Here's how the part is built. I have some questions about the finished solid (model axes, mm). A direction names the side the tool comes from. Give positions to 0.01 mm unless a question says otherwise; leave off trailing zeros. Loops run counter-clockwise (first coordinate to the right, second up) from the corner with the lowest first, then second, coordinate; pieces in that order, holes last. Notation, with made-up numbers: (21.5, 0.25) -> (73.5, 0.25) arc R22 cw to (73.5, 27.25) -> close; hole circle Ø3 at (88.5, -31.5). An arc over 180 degrees is marked (long way). Answer in a Markdown table with one row per item. Add a question column.
Item 1: If we section it at B-B (y = 0): Write out the boundary of the cut face in (x, z).
Item 2: If we section it at C-C (z = 10.5): Write out the boundary of the cut face in (x, y).
Item 3: If we section it at A-A (x = 0): Write out the boundary of the cut face in (y, z), then the cut area to 3 significant figures.
Item 4: For P1, Ø2, axis at y = 2.5, z = 50, coming from the -X side; P2, Ø1, axis at x = -2, y = 7, coming from the +Z side; P3, Ø12, axis at x = -4.5, z = 20, coming from the +Y side; P4, Ø8, axis at x = 6.5, y = 1.5, coming from the -Z side, each with a flat end and sliding along its axis, tell me the tip position at first contact or that it passes through.
Item 5: Which directions (+Z, -Z, +X, -X, +Y, -Y) give clear straight access to the entire face, cutting with the end or side of a thin tool? Please do faces 1 (the face through (-3, 8, 8)), 2 (the face through (-6, 0, 50)), 3 (the face through (-6, 0, -20)).
Item 6: If we section it at D-D (z = -13): Write out the boundary of the cut face in (x, y).
Item 7: We'd pull the mould along X, two halves only. Please class faces 4 (the face through (0, 0, -30)), 5 (the face through (3, 8, 8)), 6 (the face through (-0.806, 6.142, 39.806)), 7 (the face through (0, 7, 8)): released by +X, released by -X, zero draft, split by the parting line, or undercut.
Item 8: If I drill on line 1 (X direction, y = 8.5, z = 7); line 2 (Y direction, x = -1.5, z = 21); line 3 (Y direction, x = 0.5, z = 4), over which ranges is the centre line in solid material (lowest first)?
```python
from build123d import *

# Parameters (mm, degrees)
SKETCH2_R               = 10
BOSS_EXTRUDE1_DEPTH     = 30
SKETCH5_R               = 6
BOSS_EXTRUDE3_DEPTH     = 30
CHAMFER2_SIZE           = 10
CUT_EXTRUDE1_DEPTH      = 25
CUT_EXTRUDE1_DEPTH_BACK = 34.166247904
SKETCH3_W               = 6
SKETCH3_H               = 6
BOSS_EXTRUDE4_START     = 60
SKETCH5_3_R             = 6
BOSS_EXTRUDE4_DEPTH     = 30
CHAMFER3_SIZE           = 10


with BuildPart() as part:
    # Sketch2 → Boss-Extrude1 (new body)
    with BuildSketch(Plane.XY):
        Circle(SKETCH2_R)
    extrude(amount=BOSS_EXTRUDE1_DEPTH)

    # Sketch5 → Boss-Extrude3 (add)
    with BuildSketch(Plane.XY):
        Circle(SKETCH5_R)
    extrude(amount=-BOSS_EXTRUDE3_DEPTH)

    # Chamfer2
    # the kernel refuses this chamfer: 10 mm, written as the material it adds along each edge
    with BuildSketch(Plane(origin=(0, 0, 0), x_dir=(1, 0, 0), z_dir=(0, -1, 0))) as chamfer2_piece_1_section:
        Polygon((6 + CHAMFER2_SIZE, 0), (6, -CHAMFER2_SIZE), (6, 0), align=None)
    chamfer2_piece_1 = revolve(axis=Axis((0, 0, 0), (0, 0, 1)), mode=Mode.PRIVATE)
    chamfer2_piece_1 = chamfer2_piece_1 & Plane(origin=(0, 0, -8.05698811), x_dir=(1, 0, 0), z_dir=(0, 0, -1)) * Cylinder(10, 64, mode=Mode.PRIVATE)
    add(chamfer2_piece_1)

    # Sketch3 → Cut-Extrude1 (cut, two sides: drawn at the far end of the back side and taken through both)
    with BuildSketch(Plane.XY.offset(-CUT_EXTRUDE1_DEPTH_BACK)):
        with Locations((0, 10)):
            Rectangle(SKETCH3_W, SKETCH3_H)
    extrude(amount=CUT_EXTRUDE1_DEPTH + CUT_EXTRUDE1_DEPTH_BACK, mode=Mode.SUBTRACT)

    # Sketch5<3> → Boss-Extrude4 (add)
    with BuildSketch(Plane.XY.offset(BOSS_EXTRUDE4_START)):
        Circle(SKETCH5_3_R)
    extrude(amount=-BOSS_EXTRUDE4_DEPTH)

    # Chamfer3
    # the kernel refuses this chamfer: 10 mm, written as the material it adds along each edge
    with BuildSketch(Plane(origin=(0, 0, 30), x_dir=(1, 0, 0), z_dir=(0, -1, 0))) as chamfer3_piece_1_section:
        Polygon((6 + CHAMFER3_SIZE, 0), (6, CHAMFER3_SIZE), (6, 0), align=None)
    chamfer3_piece_1 = revolve(axis=Axis((0, 0, 30), (0, 0, 1)), mode=Mode.PRIVATE)
    chamfer3_piece_1 = chamfer3_piece_1 & Plane(origin=(0, 0, 38.05698811), x_dir=(1, 0, 0), z_dir=(0, 0, -1)) * Cylinder(10, 64, mode=Mode.PRIVATE)
    add(chamfer3_piece_1)


solid = part.part
```
Recorded:
| question | item | result |
|---|---|---|
| 1 | outline | (-10, -6) -> (-6, -10) -> (-6, -30) -> (6, -30) -> (6, -10) -> (10, -6) -> (10, 36) -> (6, 40) -> (6, 60) -> (-6, 60) -> (-6, 40) -> (-10, 36) -> close |
| 2 | outline | (-3, 7) -> (-3, 9.54) arc R10 ccw (long way) to (3, 9.54) -> (3, 7) -> close |
| 3 | outline | (-10, -6) -> (-6, -10) -> (-6, -30) -> (6, -30) -> (6, -10) -> (7, -9) -> (7, 25) -> (10, 25) -> (10, 36) -> (6, 40) -> (6, 60) -> (-6, 60) -> (-6, 40) -> (-10, 36) -> close |
| 3 | area | 1,350 mm^2 |
| 4 | P1 | stops at x = -5.81 |
| 4 | P2 | stops at z = 39.22 |
| 4 | P3 | stops at y = 9.93 |
| 4 | P4 | stops at z = -30 |
| 5 | face 1 | -Z, +Y |
| 5 | face 2 | +Z |
| 5 | face 3 | -Z |
| 6 | outline | circle Ø12 at (0, 0) |
| 7 | face 4 | zero draft |
| 7 | face 5 | undercut |
| 7 | face 6 | split by the parting line |
| 7 | face 7 | undercut |
| 8 | line 1 | x = -5.27 to -3, 3 to 5.27 |
| 8 | line 2 | y = -9.89 to 7 |
| 8 | line 3 | y = -9.99 to 7 |
